The listing builds one solid part. Answer for the finished solid, in the listing's coordinates (mm). Coordinates: 2 decimals unless noted, no trailing zeros. Order: outer loops, then holes, each group sorted by start corner. A loop starts at its lowest first (then second) coordinate and runs counter-clockwise, first axis right, second up. Notation, with made-up numbers: (62, 49.25) -> (119, 49.25) arc R27 cw to (119, 72.25) -> close; hole circle Ø1 at (-14.75, 86.25). An arc over 180 degrees is marked (long way). Answer in a Markdown table with one row per item.
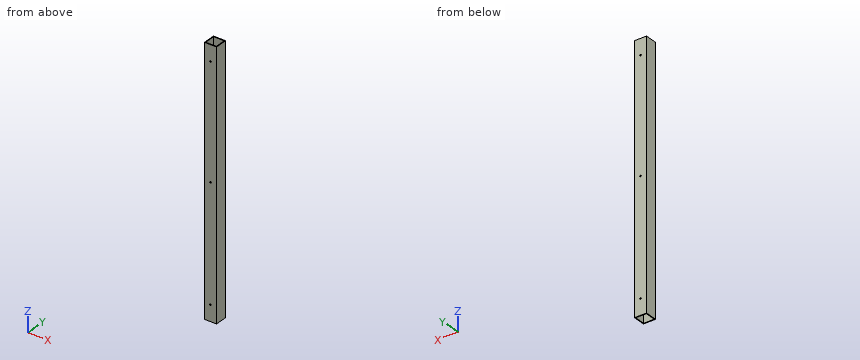
```python
from build123d import *

# Parameters (mm, degrees)
SKETCH1_W           = 50.8
SKETCH1_H           = 50.8
SKETCH1_W_2         = 44.45
SKETCH1_H_2         = 44.45
BOSS_EXTRUDE1_DEPTH = 1098.55
SKETCH2_R           = 3.302
CUT_EXTRUDE1_DEPTH  = 50.8


with BuildPart() as part:
    # Sketch1 → Boss-Extrude1 (new body)
    with BuildSketch(Plane.XY):
        with Locations((2339.531183146, 25.4)):
            Rectangle(SKETCH1_W, SKETCH1_H)
        with Locations((2339.531183146, 25.4)):
            Rectangle(SKETCH1_W_2, SKETCH1_H_2, mode=Mode.SUBTRACT)
    extrude(amount=BOSS_EXTRUDE1_DEPTH)

    # Sketch2 → Cut-Extrude1 (cut)
    with BuildSketch(Plane(origin=(0, 50.8, 0), x_dir=(1, 0, 0), z_dir=(0, 1, 0))):
        with Locations((2339.531183146, -552.45)):
            Circle(SKETCH2_R)
        with Locations((2339.531183146, -1031.875)):
            Circle(SKETCH2_R)
        with Locations((2339.531183146, -66.802)):
            Circle(SKETCH2_R)
    extrude(amount=-CUT_EXTRUDE1_DEPTH, mode=Mode.SUBTRACT)


solid = part.part
```
(1) A cutting plane is placed at A-A, the plane z = 800. Determine the outline of the cut face in (x, y) (3 decimals), then the cut area to 3 significant figures.
Check values:
| item | result |
|---|---|
| outline | (2314.131, 0) -> (2364.931, 0) -> (2364.931, 50.8) -> (2314.131, 50.8) -> close; hole (2317.306, 3.175) -> (2361.756, 3.175) -> (2361.756, 47.625) -> (2317.306, 47.625) -> close |
| area | 605 mm² |
(2) A flat-ended cylindrical pin translates along its axis: pin 1 (5.5 mm diameter, centred on x = 2339.53, z = 552.45, fed in from -Y). Find the tip coordinate at first contact, or state that the pin passes through.
Check values:
| item | result |
|---|---|
| pin 1 | through |
(3) Find the intervals of material crossed by line 1 along Y through (x, z) = (2346, 113) (3 decimals); line 2 along X through (y, z) = (15, 1042.5); line 3 along X through (y, z) = (48, 552), in increasing order. Write a range as from..to.
Check values:
| item | result |
|---|---|
| line 1 | 0..3.175, 47.625..50.8 |
| line 2 | 2314.13..2317.31, 2361.76..2364.93 |
| line 3 | 2314.13..2336.26, 2342.8..2364.93 |
(4) A cutting plane is placed at B-B, the plane y = 23. Determine the outline of the cut face in (x, z), then the cut area to 3 significant figures.
Check values:
| item | result |
|---|---|
| outline | (2314.13, 0) -> (2317.31, 0) -> (2317.31, 1098.55) -> (2314.13, 1098.55) -> close; (2361.76, 0) -> (2364.93, 0) -> (2364.93, 1098.55) -> (2361.76, 1098.55) -> close |
| area | 6,980 mm² |
